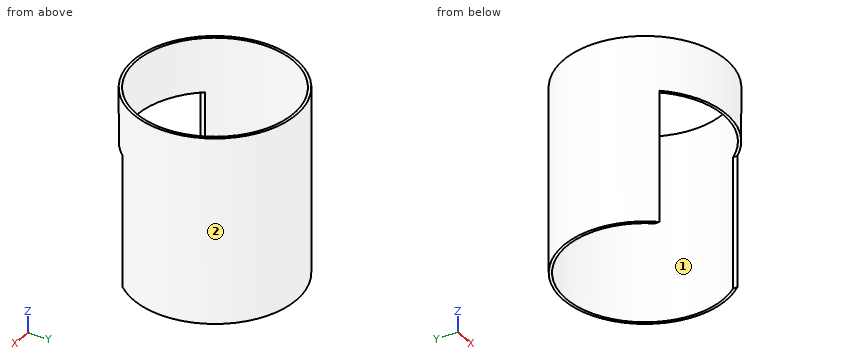
from build123d import *

# Parameters (mm, degrees)
SKETCH004_W      = 86
SKETCH004_H      = 92
EXTRUDE005_DEPTH = 68.155048
TUBE_R           = 57.15
TUBE_R_2         = 55.15
TUBE_DEPTH       = 130


with BuildPart() as holeboiler:
    # Sketch004 → Extrude005 (new body)
    with BuildSketch(Plane.XZ):
        with Locations((0, 66)):
            Rectangle(SKETCH004_W, SKETCH004_H)
    extrude(amount=EXTRUDE005_DEPTH)


with BuildPart() as cut:
    # Tube → Tube (new body)
    with BuildSketch(Plane.XY.offset(20)):
        Circle(TUBE_R)
        Circle(TUBE_R_2, mode=Mode.SUBTRACT)
    extrude(amount=TUBE_DEPTH)

    # Cut: cut HoleBoiler
    add(holeboiler.part, mode=Mode.SUBTRACT)


solid = cut.part
Source: CAD feature listing. Evaluate the final solid. Frame: model axes, mm. Face numbers are marked on the shaded views. Give positions to 0.01 mm unless a question says otherwise; leave off trailing zeros. Write each loop counter-clockwise with the first axis right and the second up, starting at its lowest first coordinate (ties: lowest second). Pieces come first, ordered by that corner, then holes. Notation, with made-up numbers: M -0.5,52.25 L 45.5,52.25 A19 ccw 45.5,77.25 Z; hole C 67.25,-38 d4. An arc over 180 degrees is marked long. Return JSON: item names as keys, results as strings. Group by question number.
1) Cut plane C-C, the plane z = 44.5. Output: boundary loops of the cut face in (x, y).
2) Cut plane B-B, the plane y = 0. Output: boundary loops of the cut face in (x, z).
3) Pin query (flat end, axial travel): P1, Ø5, axis at y = 43.5, z = 132.5, coming from the +X side; P2, Ø0.9, axis at y = -37, z = 53.5, coming from the +X side; P3, Ø4, axis at x = -27.5, z = 48, coming from the -Y side; P4, Ø18, axis at x = 10.5, y = -40.5, coming from the -Z side. Return the tip coordinate at first contact, or that it passes through.
4) Cut plane A-A, the plane x = 0. Output: boundary loops of the cut face in (y, z).
5) Pull-direction query (X, two-part tool) for the marked faces 1 and 2; classes: pulls with the +X half, pulls with the -X half, needs draft (parallel to the pull), parting line crosses it, or undercut.
6) Material intervals for line 1 along X through (y, z) = (0, 66); line 2 along Y through (x, z) = (0, 66); line 3 along X through (y, z) = (45, 91.5), sorted ascending. Write a range as [from, to].
Recorded:
{
 "1": {"outline": "M -43,-37.64 L -43,-34.53 A55.15 cw long 43,-34.53 L 43,-37.64 A57.15 ccw long Z"},
 "2": {"outline": "M -57.15,20 L -55.15,20 L -55.15,150 L -57.15,150 Z; M 55.15,20 L 57.15,20 L 57.15,150 L 55.15,150 Z"},
 "3": {"P1": "stops at x = 39.81", "P2": "stops at x = 43.93", "P3": "stops at y = 46.6", "P4": "passes through"},
 "4": {"outline": "M -57.15,112 L -55.15,112 L -55.15,150 L -57.15,150 Z; M 55.15,20 L 57.15,20 L 57.15,150 L 55.15,150 Z"},
 "5": {"face 1": "undercut", "face 2": "parting line crosses it"},
 "6": {"line 1": "x = [-57.15, -55.15], [55.15, 57.15]", "line 2": "y = [55.15, 57.15]", "line 3": "x = [-35.23, -31.88], [31.88, 35.23]"}
}
